Source: CAD feature listing. Evaluate the final solid. Frame: model axes, mm. Face numbers are marked on the shaded views. A direction names the side the tool comes from. Give positions to 0.01 mm unless a question says otherwise; leave off trailing zeros. Loops run counter-clockwise (first coordinate to the right, second up) from the corner with the lowest first, then second, coordinate; pieces in that order, holes last.
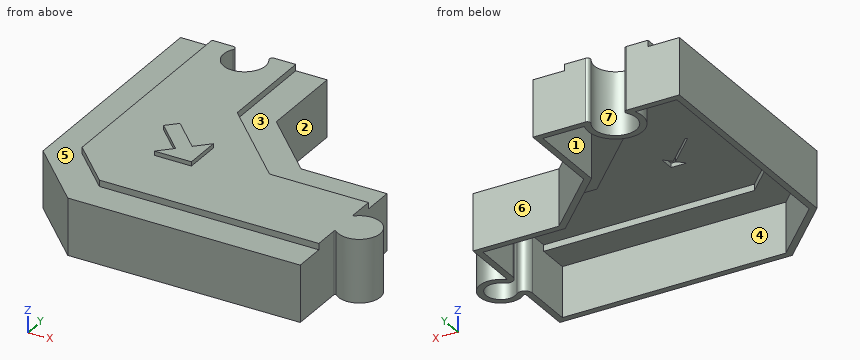
```python
from build123d import *

# Parameters (mm, degrees)
BOSS_EXTRU_1_DEPTH      = 30
BOSS_EXTRU_2_DEPTH      = 30
ENL_V_MAT_EXTRU_1_DEPTH = 152.492574075
ESQUISSE4_R             = 10
ENL_V_MAT_EXTRU_2_DEPTH = 50
ESQUISSE5_R             = 10
BOSS_EXTRU_3_DEPTH      = 30
ENL_V_MAT_EXTRU_3_DEPTH = 3
BOSS_EXTRU_4_DEPTH      = 2
CONG_2_R                = 0.5
CONG_3_R                = 1.5
COQUE1_DEPTH            = 24
COQUE1_START            = 24
COQUE1_2_DEPTH          = 3
COQUE1_START_2          = 27
COQUE1_3_DEPTH          = 2


# Read off the part's stored shape, not the designer's step: Coque1
with BuildPart() as part:
    # Esquisse1 → Boss.-Extru.1 (new body)
    with BuildSketch(Plane.XY):
        Polygon((-35, 105), (35, 105), (35, 35), (105, 35), (105, -35), (-35, -35), align=None)
    extrude(amount=BOSS_EXTRU_1_DEPTH)

    # Esquisse2 → Boss.-Extru.2 (add)
    with BuildSketch(Plane.XY.offset(30)):
        Polygon((35, 63.969429202), (63.969429202, 35), (35, 35), align=None)
    extrude(amount=-BOSS_EXTRU_2_DEPTH)

    # Esquisse3 → Enlèv. mat.-Extru.1 (cut, through all)
    with BuildSketch(Plane.XY.offset(30)):
        Polygon((-35, -35), (-6.009429202, -35), (-35, -6.009429202), align=None)
    extrude(amount=-ENL_V_MAT_EXTRU_1_DEPTH, mode=Mode.SUBTRACT)

    # Esquisse4 → Enlèv. mat.-Extru.2 (cut)
    with BuildSketch(Plane.XY.offset(30)):
        with Locations((0, 97.5)):
            Circle(ESQUISSE4_R)
    extrude(amount=-ENL_V_MAT_EXTRU_2_DEPTH, mode=Mode.SUBTRACT)

    # Esquisse5 → Boss.-Extru.3 (add, through all)
    with BuildSketch(Plane.XY.offset(30)):
        with Locations((112.5, 0)):
            Circle(ESQUISSE5_R)
    extrude(amount=-BOSS_EXTRU_3_DEPTH)

    # Esquisse7 → Enlèv. mat.-Extru.3 (cut)
    with BuildSketch(Plane.XY.offset(30)):
        Polygon((20, 57.756225766), (20, 105), (35, 105), (35, 63.969429202), (63.969429202, 35), (105, 35), (105, 20), (57.756225766, 20), align=None)
        Polygon((0.203774234, -20), (105, -20), (105, -35), (-6.009429202, -35), (-35, -6.009429202), (-35, 105), (-20, 105), (-20, 0.203774234), align=None)
    extrude(amount=-ENL_V_MAT_EXTRU_3_DEPTH, mode=Mode.SUBTRACT)

    # Esquisse8 → Boss.-Extru.4 (add)
    with BuildSketch(Plane.XY.offset(30)):
        Polygon((1.267051582, 29.97688251), (6.21679905, 34.926629979), (20.358934674, 20.784494355), (26.736260006, 27.161819687), (26.736260006, 9.457421554), (9.031861873, 9.457421554), (15.409187205, 15.834746887), align=None)
    extrude(amount=BOSS_EXTRU_4_DEPTH)

    # Congé2
    cong_2_edges = [part.edges().sort_by_distance(p)[0] for p in [
        (105, -6.614378278, 15),
        (105, 6.614378278, 15),
    ]]
    fillet(cong_2_edges, radius=CONG_2_R)

    # Congé3
    cong_3_edges = [part.edges().sort_by_distance(p)[0] for p in [
        (6.614378278, 105, 15),
        (-6.614378278, 105, 15),
    ]]
    fillet(cong_3_edges, radius=CONG_3_R)

    # Coque1 outline → Coque1 (cut)
    with BuildSketch(Plane.XY):
        with BuildLine():
            Line((-32, 102), (-32, -4.766788515))
            Line((-32, -4.766788515), (-4.766788515, -32))
            Line((-4.766788515, -32), (102, -32))
            Line((102, -32), (102, -7.826237921))
            ThreePointArc((102, -7.826237921), (104.071130983, -4.631189669), (107.833333333, -5.217491947))
            ThreePointArc((107.833333333, -5.217491947), (119.5, 0), (107.833333333, 5.217491947))
            ThreePointArc((107.833333333, 5.217491947), (104.071130983, 4.631189669), (102, 7.826237921))
            Line((102, 7.826237921), (102, 32))
            Line((102, 32), (62.726788515, 32))
            Line((62.726788515, 32), (32, 62.726788515))
            Line((32, 62.726788515), (32, 102))
            Line((32, 102), (12.196310918, 102))
            ThreePointArc((12.196310918, 102), (0, 84.5), (-12.196310918, 102))
            Line((-12.196310918, 102), (-32, 102))
        make_face()
    extrude(amount=COQUE1_DEPTH, mode=Mode.SUBTRACT)

    # Coque1 2 outline → Coque1 2 (cut)
    with BuildSketch(Plane.XY.offset(COQUE1_START)):
        with BuildLine():
            Line((-12.196310918, 102), (-17, 102))
            Line((-17, 102), (-17, 1.446414921))
            Line((-17, 1.446414921), (1.446414921, -17))
            Line((1.446414921, -17), (102, -17))
            Line((102, -17), (102, -7.826237921))
            ThreePointArc((102, -7.826237921), (104.071130983, -4.631189669), (107.833333333, -5.217491947))
            ThreePointArc((107.833333333, -5.217491947), (119.5, 0), (107.833333333, 5.217491947))
            ThreePointArc((107.833333333, 5.217491947), (104.071130983, 4.631189669), (102, 7.826237921))
            Line((102, 7.826237921), (102, 17))
            Line((102, 17), (56.513585079, 17))
            Line((56.513585079, 17), (17, 56.513585079))
            Line((17, 56.513585079), (17, 102))
            Line((17, 102), (12.196310918, 102))
            ThreePointArc((12.196310918, 102), (0, 84.5), (-12.196310918, 102))
        make_face()
    extrude(amount=COQUE1_2_DEPTH, mode=Mode.SUBTRACT)

    # Coque1 3 outline → Coque1 3 (cut)
    with BuildSketch(Plane.XY.offset(COQUE1_START_2)):
        Polygon((5.509692269, 29.97688251), (19.651827893, 15.834746887), (16.27450256, 12.457421554), (23.736260006, 12.457421554), (23.736260006, 19.919179), (20.358934674, 16.541853668), (6.21679905, 30.683989291), align=None)
    extrude(amount=COQUE1_3_DEPTH, mode=Mode.SUBTRACT)


solid = part.part
```
(1) Section B-B, the plane y = 97.5. Return the cut outline in (x, z), then the cut area to 3 significant figures.
A:
outline: (-35, 0) - (-32, 0) - (-32, 24) - (-17, 24) - (-17, 27) - (-13, 27) - (-13, 0) - (-10, 0) - (-10, 30) - (-20, 30) - (-20, 27) - (-35, 27) - close; (10, 0) - (13, 0) - (13, 27) - (17, 27) - (17, 24) - (32, 24) - (32, 0) - (35, 0) - (35, 27) - (20, 27) - (20, 30) - (10, 30) - close
area: 474 mm2
(2) Section A-A, the plane y = 76.5. Return the cut outline in (x, z).
A:
outline: (-35, 0) - (-32, 0) - (-32, 24) - (-17, 24) - (-17, 27) - (17, 27) - (17, 24) - (32, 24) - (32, 0) - (35, 0) - (35, 27) - (20, 27) - (20, 30) - (-20, 30) - (-20, 27) - (-35, 27) - close
(3) First-contact query: pin 1 (1 mm diameter, centred on x = 15, z = 31, fed in from -Y); pin 2 (2 mm diameter, centred on y = 31.5, z = 22.5, fed in from +X); pin 3 (23 mm diameter, centred on x = 0, y = 97.5, fed in from -Z); pin 4 (1.5 mm diameter, centred on x = 57, z = 25.5, fed in from +Y). Flat tips, straight axial feed; report the tip coordinate or a pass-through.
A:
pin 1: stops at y = 9.46
pin 2: stops at x = 105
pin 3: stops at z = 0
pin 4: stops at y = 42.72
(4) Section D-D, the plane x = 50.5. Return the cut outline in (y, z), then the cut area to 3 significant figures.
A:
outline: (-35, 0) - (-32, 0) - (-32, 24) - (-17, 24) - (-17, 27) - (23.01, 27) - (23.01, 24) - (44.23, 24) - (44.23, 0) - (48.47, 0) - (48.47, 27) - (27.26, 27) - (27.26, 30) - (-20, 30) - (-20, 27) - (-35, 27) - close
area: 446 mm2
(5) Ray query, line 1 along X through (y, z) = (97, 7); line 2 along Y through (x, z) = (112, 14); line 3 along Y through (x, z) = (69, 16.5). Return the intervals inside material, ascending.
A:
line 1: x = -35 to -32, -12.99 to -9.99, 9.99 to 12.99, 32 to 35
line 2: y = -9.99 to -6.98, 6.98 to 9.99
line 3: y = -35 to -32, 32 to 35
(6) Mould query, pull axis X, two halves, no side actions, for the marked faces 1, 2 and 3. Classes: pulls with the +X half, pulls with the -X half, needs draft (parallel to the pull), parting line crosses it, or undercut.
A:
face 1: undercut
face 2: pulls with the +X half
face 3: needs draft
(7) Reachability of the marked faces 4, 5, 6 and 7 from +Z, -Z, +X, -X, +Y, -Y: full face, straight path, thin tool, end or side. Return the list, or none.
A:
face 4: -Z
face 5: +Z, -X, -Y
face 6: +Z, -Z, +X, +Y
face 7: +Z, -Z
